Build history of the part. All positions in model axes, mm. A direction names the side the tool comes from. Give positions to 0.01 mm unless a question says otherwise; leave off trailing zeros. Order: outer loops, then holes, each group sorted by start corner. A loop starts at its lowest first (then second) coordinate and runs counter-clockwise, first axis right, second up. Notation, with made-up numbers: (82.5, 0.5) - (89.5, 0.5) arc R36 ccw to (89.5, 37.5) - close; hole circle Ø5 at (-32, -13). An arc over 180 degrees is marked (long way). Use a Markdown table: item, result.
from build123d import *

# Parameters (mm, degrees)
SKETCH1_R           = 12.5
BOSS_EXTRUDE1_DEPTH = 25.65
BOSS_EXTRUDE2_DEPTH = 16.2
SKETCH2_3_R         = 4
SKETCH2_3_R_2       = 2
BOSS_EXTRUDE3_DEPTH = 6.5
CUT_EXTRUDE2_DEPTH  = 17


with BuildPart() as part:
    # Sketch1 → Boss-Extrude1 (new, symmetric)
    with BuildSketch(Plane(origin=(0, 0, 0), x_dir=(1, 0, 0), z_dir=(0, 1, 0))):
        with Locations(Location((0, 0, 0), (0, 0, 270))):
            Circle(SKETCH1_R)
    extrude(amount=BOSS_EXTRUDE1_DEPTH, both=True)

    # Sketch2 → Boss-Extrude2 (add)
    with BuildSketch(Plane(origin=(0, 25.65, 0), x_dir=(1, 0, 0), z_dir=(0, 1, 0))):
        with BuildLine():
            ThreePointArc((1.5612495, 1.25), (0, 2), (-1.5612495, 1.25))
            Line((-1.5612495, 1.25), (1.5612495, 1.25))
        make_face()
        with BuildLine():
            Line((1.5612495, 1.25), (-1.5612495, 1.25))
            ThreePointArc((-1.5612495, 1.25), (-0.662382443, -1.887127314), (2, 0))
            ThreePointArc((2, 0), (1.887127314, 0.662382443), (1.5612495, 1.25))
        make_face()
    extrude(amount=BOSS_EXTRUDE2_DEPTH)

    # Sketch2<3> → Boss-Extrude3 (add)
    with BuildSketch(Plane(origin=(0, 25.65, 0), x_dir=(1, 0, 0), z_dir=(0, 1, 0))):
        with Locations(Location((0, 0, 0), (0, 0, 90))):
            Circle(SKETCH2_3_R)
        with Locations(Location((0, 0, 0), (0, 0, 270))):
            Circle(SKETCH2_3_R_2, mode=Mode.SUBTRACT)
    extrude(amount=BOSS_EXTRUDE3_DEPTH)

    # Sketch2<4> → Cut-Extrude2 (cut)
    with BuildSketch(Plane(origin=(0, 25.65, 0), x_dir=(1, 0, 0), z_dir=(0, 1, 0))):
        with BuildLine():
            ThreePointArc((1.5612495, 1.25), (0, 2), (-1.5612495, 1.25))
            Line((-1.5612495, 1.25), (1.5612495, 1.25))
        make_face()
    extrude(amount=CUT_EXTRUDE2_DEPTH, mode=Mode.SUBTRACT)


solid = part.part
1) Wall check: line 1 (Y direction, x = -9, z = -2); line 2 (Z direction, x = 2.25, y = 19.5); line 3 (X direction, y = -13.5, z = -6). Give the ranges that are in metal, low to high. Write a range as from..to.
Computed:
| item | result |
|---|---|
| line 1 | y = -25.65..25.65 |
| line 2 | z = -12.3..12.3 |
| line 3 | x = -10.97..10.97 |
2) Tool access for faces 4 (the flat face through (3, 25.65, -3)), 5 (the flat face through (0, -25.65, 0)): list every direction of +Z, -Z, +X, -X, +Y, -Y with a clear straight run to the whole face (end or side of a thin tool).
Computed:
| item | result |
|---|---|
| face 4 | +Y |
| face 5 | +Z, -Z, +X, -X, -Y |
3) Slice it at C-C (y = -3.5). Write the cut outline in (x, z).
Computed:
| item | result |
|---|---|
| outline | circle Ø25 at (0, 0) |
4) Slice it at B-B (y = 29.5). Write the cut outline in (x, z).
Computed:
| item | result |
|---|---|
| outline | circle Ø8 at (0, 0); hole (-1.56, -1.25) arc R2 ccw to (1.56, -1.25) - close |
5) Two-plate mould, pull along Z, no slides. Class faces 1 (the cylindrical face through (3.905, 28.854, 0.867)), 2 (the flat face through (0, 34, -1.25)), 3 (the flat face through (0, 41.85, 0)): +Z half, -Z half, draft (parallel to the pull), parting line (faces both ways), or undercut.
Computed:
| item | result |
|---|---|
| face 1 | parting line |
| face 2 | undercut |
| face 3 | draft |
6) Slice it at A-A (x = 0). Write the cut outline in (y, z), and give its area (3 significant figures).
Computed:
| item | result |
|---|---|
| outline | (-25.65, -12.5) - (25.65, -12.5) - (25.65, -4) - (32.15, -4) - (32.15, -2) - (25.65, -2) - (25.65, -1.25) - (41.85, -1.25) - (41.85, 2) - (32.15, 2) - (32.15, 4) - (25.65, 4) - (25.65, 12.5) - (-25.65, 12.5) - close |
| area | 1,360 mm² |
7) Slice it at D-D (z = 11.25). Write the cut outline in (x, y), and give its area (3 significant figures).
Computed:
| item | result |
|---|---|
| outline | (-5.45, -25.65) - (5.45, -25.65) - (5.45, 25.65) - (-5.45, 25.65) - close |
| area | 559 mm² |
8) Pin check, flat tips, straight feed: P1, Ø5, axis at y = 27, z = 4, coming from the -X side; P2, Ø6, axis at x = -7, y = 14, coming from the +Z side; P3, Ø3, axis at y = 24.5, z = -7, coming from the +X side (3 decimals). Stop position of each tip, or through.
Computed:
| item | result |
|---|---|
| P1 | stops at x = -12.36 |
| P2 | stops at z = 11.84 |
| P3 | stops at x = 11.225 |
